Autodesk Inventor part; units mm, degrees
ref_plane "YZ Plane" through (0, 0, 0) normal (1, 0, 0) x (0, 1, 0)
ref_plane "XZ Plane" through (0, 0, 0) normal (0, 1, 0) x (-1, 0, 0)
ref_plane "XY Plane" through (0, 0, 0) normal (0, 0, 1) x (1, 0, 0)
sketch "Skizze1" plane through (0, 0, 0) normal (1, 0, 0) x (0, 1, 0)
  line L0 (-44.5, -5.5) -> (40.5, -5.5)
  line L1 (44.5, -9.5) -> (-44.5, -9.5)
  line L2 (-44.5, -9.5) -> (-44.5, -5.5)
  line L3 (40.5, -5.5) -> (40.5, 9.5)
  line L4 (40.5, 9.5) -> (44.5, 9.5)
  line L5 (44.5, 9.5) -> (44.5, -9.5)
  point P0 (0, 0)
  point P1 (44.5, 0)
  point P2 (0, -9.5)
  dimension "d0" = 4
  dimension "d2" = 4
  dimension "d3" = 19
  dimension "d6" = 89
extrude "Extrusion1" add sketch "Skizze1" along normal mid plane 54
properties part number "Platinenhalter-einzeln"
Input: part model. Units: mm. Frame: model coordinates. A direction names the side the tool comes from. Give positions to 0.01 mm unless a question says otherwise; leave off trailing zeros. Order: outer loops, then holes, each group sorted by start corner. A loop starts at its lowest first (then second) coordinate and runs counter-clockwise, first axis right, second up. Notation, with made-up numbers: M 13,-7.5 L 33,-7.5 A17 ccw 33,24.5 Z; hole C 65.5,73.25 d4. An arc over 180 degrees is marked long. Answer as a JSON object with one key per item and string values.
1. Reachability of faces 1 (the flat face through (0, 42, 9.5)), 2 (the flat face through (0, 40.5, 2)) from +Z, -Z, +X, -X, +Y, -Y: full face, straight path, thin tool, end or side. Return the list, or none.
Result sheet:
{"face 1": "+Z, +X, -X, +Y, -Y", "face 2": "+Z, +X, -X, -Y"}
2. Ray query, line 1 (Y direction, x = 16, z = 8.25); line 2 (Z direction, x = -6, y = 30). Return the intervals inside material, ascending. Write a range as [from, to].
Result sheet:
{"line 1": "[40.5, 44.5]", "line 2": "[-9.5, -5.5]"}
3. Cut plane A-A, the plane x = 3. Output: boundary loops of the cut face in (y, z).
Result sheet:
{"outline": "M -44.5,-9.5 L 44.5,-9.5 L 44.5,9.5 L 40.5,9.5 L 40.5,-5.5 L -44.5,-5.5 Z"}
4. Cut plane B-B, the plane y = 26. Output: boundary loops of the cut face in (x, z), and give its area (3 significant figures).
Result sheet:
{"outline": "M -27,-9.5 L 27,-9.5 L 27,-5.5 L -27,-5.5 Z", "area": "216 mm²"}
5. First-contact query: P1, Ø3, axis at x = -20.5, y = -11.5, coming from the +Z side; P2, Ø7.5, axis at x = 8.5, z = 3, coming from the -Y side; P3, Ø10, axis at y = -5.5, z = 2, coming from the +X side. Flat tips, straight axial feed; report the tip coordinate or a pass-through.
Result sheet:
{"P1": "z = -5.5", "P2": "y = 40.5", "P3": "through"}
6. Cut plane C-C, the plane z = -3.5. Output: boundary loops of the cut face in (x, y).
Result sheet:
{"outline": "M -27,40.5 L 27,40.5 L 27,44.5 L -27,44.5 Z"}
